Input: dimensioned drawing with shaded views. Units: mm. Origin: part minimum x, y, z. A direction names the side the tool comes from. Round coordinates to 2 decimals unless told otherwise and drop trailing zeros. Loops run counter-clockwise (first coordinate to the right, second up) from the corner with the lowest first, then second, coordinate; pieces in that order, holes last. Notation, with made-up numbers: M -13,88.5 L 6,88.5 A13 cw 6,113.5 Z; hole C 46,81 d1. An arc over 180 degrees is marked long. Put each result on its own line as item: value. Start each with the question number.
1) Draft query along Y for the marked faces 3, 4 and 5. Return one class per face: +Y half, -Y half, draft (parallel to the pull), parting line (faces both ways), or undercut.
2) Line query: probe 1 along Y at (x, z) = (5, 2.25); probe 2 along Y at (x, z) = (6.25, 2.75); probe 3 along X at (y, z) = (6.5, 8). Output: solid intervals per line, ascending.
3) Reachability of the marked faces 1 and 2 from +Z, -Z, +X, -X, +Y, -Y: full face, straight path, thin tool, end or side. Return the list, or none.
4) Section C-C on y = 45. Output: boundary loops of the cut face in (x, z), plus the area to 3 significant figures.
5) Section B-B on x = 5. Output: boundary loops of the cut face in (y, z), plus the area to 3 significant figures.
6) Section D-D on x = 7. Output: boundary loops of the cut face in (y, z), plus the area to 3 significant figures.
7) Section A-A on z = 5. Output: boundary loops of the cut face in (x, y).
8) Pin query (flat end, axial travel): pin 1 (4 mm diameter, centred on y = 37, z = 2, fed in from +X); pin 2 (2.5 mm diameter, centred on x = 5, y = 45, fed in from -Z); pin 3 (4 mm diameter, centred on y = 37, z = 3, fed in from +X); pin 4 (6 mm diameter, centred on x = 4, y = 35.5, fed in from -Z). Return the tip coordinate at first contact, or that it passes through.
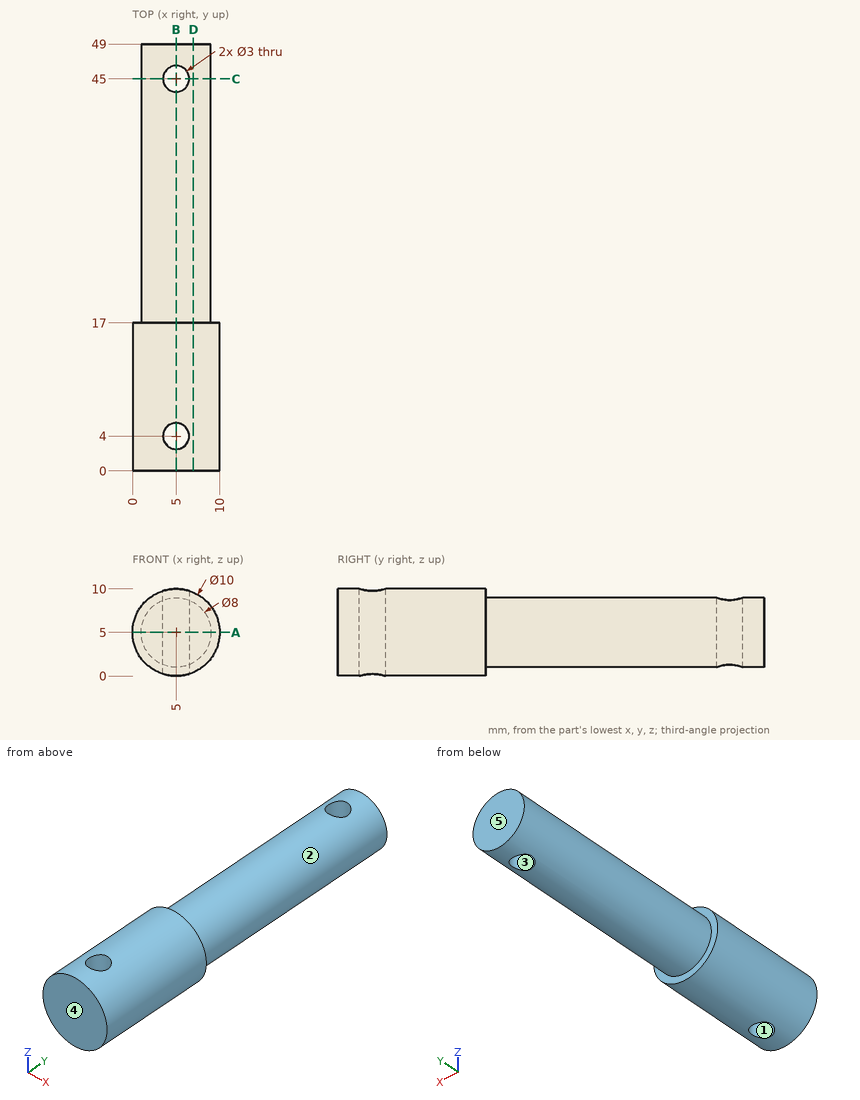
Geometry results:
1. face 3: undercut
1. face 4: -Y half
1. face 5: +Y half
2. probe 1: y = 0 to 2.5, 5.5 to 43.5, 46.5 to 49
2. probe 2: y = 0 to 3.17, 4.83 to 44.17, 45.83 to 49
2. probe 3: x = 1 to 9
3. face 1: +Z, -Z
3. face 2: +Y
4. outline: M 3.5,1.29 L 3.5,8.71 A4 ccw Z; M 6.5,1.29 A4 ccw 6.5,8.71 Z
4. area: 26.8 mm²
5. outline: M 0,0 L 2.5,0 L 2.5,10 L 0,10 Z; M 5.5,0 L 17,0 L 17,1 L 43.5,1 L 43.5,9 L 17,9 L 17,10 L 5.5,10 Z; M 46.5,1 L 49,1 L 49,9 L 46.5,9 Z
5. area: 372 mm²
6. outline: M 0,0.42 L 17,0.42 L 17,1.54 L 49,1.54 L 49,8.46 L 17,8.46 L 17,9.58 L 0,9.58 Z
6. area: 378 mm²
7. outline: M 0,0 L 10,0 L 10,17 L 9,17 L 9,49 L 1,49 L 1,17 L 0,17 Z; hole C 5,4 d3; hole C 5,45 d3
8. pin 1: stops at x = 8.87
8. pin 2: passes through
8. pin 3: stops at x = 9
8. pin 4: stops at z = 1
